Build history of the part. All positions in model axes, mm. Face numbers are marked on the shaded views. A direction names the side the tool comes from. Round coordinates to 2 decimals unless told otherwise and drop trailing zeros. Order: outer loops, then holes, each group sorted by start corner. A loop starts at its lowest first (then second) coordinate and runs counter-clockwise, first axis right, second up. Notation, with made-up numbers: (36.25, -16) - (95.25, -16) arc R26 ccw to (95.25, -2) - close; hole circle Ø3 at (51.25, 68). An arc over 180 degrees is marked (long way). Write each question's results on one line, items separated by ' | '. Start each with the question number.
```python
from build123d import *

# Parameters (mm, degrees)
BOSS_EXTRUDE1_DEPTH = 50.8
SKETCH2_R           = 12.7
CUT_EXTRUDE1_DEPTH  = 50.8
CUT_EXTRUDE2_DEPTH  = 50.8
SKETCH5_R           = 1.166747446
CUT_EXTRUDE3_DEPTH  = 7.62


with BuildPart() as part:
    # Sketch1 → Boss-Extrude1 (new body)
    with BuildSketch(Plane.XY):
        with BuildLine():
            Line((17.78, 16.984869565), (17.78, -30.259130435))
            Line((17.78, -30.259130435), (-12.7, -30.259130435))
            Line((-12.7, -30.259130435), (-12.7, 16.984869565))
            ThreePointArc((-12.7, 16.984869565), (2.54, 32.224869565), (17.78, 16.984869565))
        make_face()
    extrude(amount=BOSS_EXTRUDE1_DEPTH)

    # Sketch2 → Cut-Extrude1 (cut)
    with BuildSketch(Plane.XY.offset(50.8)):
        with Locations((2.54, 18.54261415)):
            Circle(SKETCH2_R)
    extrude(amount=-CUT_EXTRUDE1_DEPTH, mode=Mode.SUBTRACT)

    # Sketch4 → Cut-Extrude2 (cut)
    with BuildSketch(Plane(origin=(17.78, 0, 0), x_dir=(0, 0, -1), z_dir=(1, 0, 0))):
        Polygon((-47.247044422, 3.453714402), (-2.664546428, 3.453714402), (-47.247044422, -10.657322195), align=None)
        Polygon((-47.247044422, -13.645405957), (-2.664546428, 0.46563064), (-2.664546428, -25.553882978), (-47.247044422, -25.553882978), align=None)
    extrude(amount=-CUT_EXTRUDE2_DEPTH, mode=Mode.SUBTRACT)

    # Sketch5 → Cut-Extrude3 (cut)
    with BuildSketch(Plane(origin=(0, -30.259130435, 0), x_dir=(-1, 0, 0), z_dir=(0, -1, 0))):
        with Locations(Location((7.62, -12.7, 0), (0, 0, 90))):
            Circle(SKETCH5_R)
        with Locations(Location((7.62, -38.1, 0), (0, 0, 90))):
            Circle(SKETCH5_R)
        with Locations(Location((-12.7, -38.1, 0), (0, 0, 90))):
            Circle(SKETCH5_R)
        with Locations(Location((-12.7, -12.7, 0), (0, 0, 90))):
            Circle(SKETCH5_R)
    extrude(amount=-CUT_EXTRUDE3_DEPTH, mode=Mode.SUBTRACT)


solid = part.part
```
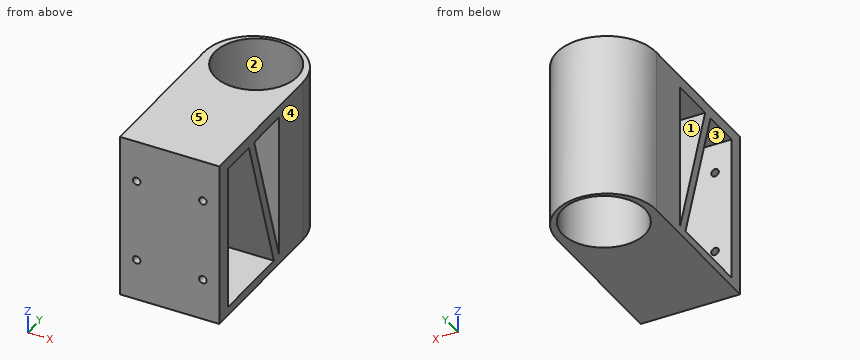
1. Cut at B-B (x = 12.7). List the corners of the cut face in (y, z).
2. Cut at C-C (z = 43). List the corners of the cut face in (x, y), plus the area to 3 significant figures.
3. Mould opens along Z. For the marked faces 3, 4 and 5 say: pulls with the +Z half, pulls with the -Z half, needs draft (parallel to the pull), parting line crosses it, or undercut.
4. Cut at D-D (y = 14). List the corners of the cut face in (x, z).
5. Cut at A-A (x = 2.54). List the corners of the cut face in (y, z).
6. Flat gauge pins, fed straight in: pin 1 Ø15 at (x, z) = (9.5, 33.5) entering from +Y; pin 2 Ø1.5 at (x, z) = (-3, 7) entering from +Y; pin 3 Ø1.9 at (x, z) = (-7.62, 12.7) entering from -Y; pin 4 Ø3.5 at (x, z) = (12.7, 12.7) entering from +Y. Where does each tip first touch, or does it go through?
7. 3-axis set-ups, long thin cutter, end or side, ignore diameter. For the marked faces 1 and 2: which of +Z, -Z, +X, -X, +Y, -Y reach the whole face in a straight line?
8. Wall check: line 1 (Z direction, x = 2, y = -14); line 2 (Y direction, x = 2.54, z = 14); line 3 (Y direction, x = -6, z = 8.5). Give the ranges that are in metal, low to high. Write a range as from..to.
A:
1) outline: (-30.26, 0) - (10.92, 0) - (10.92, 50.8) - (-30.26, 50.8) - (-30.26, 39.27) - (-25.55, 39.27) - (-25.55, 47.25) - (-13.65, 47.25) - (0.47, 2.66) - (-25.55, 2.66) - (-25.55, 11.53) - (-30.26, 11.53) - close; (-30.26, 13.87) - (-25.55, 13.87) - (-25.55, 36.93) - (-30.26, 36.93) - close; (26.16, 0) - (28.34, 0) - (28.34, 50.8) - (26.16, 50.8) - close; hole (-10.66, 47.25) - (3.45, 2.66) - (3.45, 47.25) - close
2) outline: (-12.7, -30.26) - (17.78, -30.26) - (17.78, -25.55) - (-12.7, -25.55) - close; (-12.7, -12.3) - (17.78, -12.3) - (17.78, -9.31) - (-12.7, -9.31) - close; (-12.7, 3.45) - (17.78, 3.45) - (17.78, 16.98) arc R15.24 ccw to (-12.7, 16.98) - close; hole circle Ø25.4 at (2.54, 18.54) | area: 505 mm^2
3) face 3: undercut | face 4: needs draft | face 5: pulls with the +Z half
4) outline: (-12.7, 0) - (-9.32, 0) - (-9.32, 50.8) - (-12.7, 50.8) - close; (14.4, 0) - (17.78, 0) - (17.78, 50.8) - (14.4, 50.8) - close
5) outline: (-30.26, 0) - (5.84, 0) - (5.84, 50.8) - (-30.26, 50.8) - close; (31.24, 0) - (32.22, 0) - (32.22, 50.8) - (31.24, 50.8) - close; hole (-25.55, 2.66) - (0.47, 2.66) - (-13.65, 47.25) - (-25.55, 47.25) - close; hole (-10.66, 47.25) - (3.45, 2.66) - (3.45, 47.25) - close
6) pin 1: stops at y = 32.22 | pin 2: stops at y = 31.45 | pin 3: stops at y = -3.01 | pin 4: stops at y = 29.69
7) face 1: +X, -X | face 2: +Z, -Z
8) line 1: z = 0..2.66, 47.25..50.8 | line 2: y = -30.26..-25.55, -3.12..-0.13, 3.45..5.84, 31.24..32.22 | line 3: y = -30.26..-25.55, -1.38..1.61, 3.45..9.14, 27.94..29.61
